Read the model definition and answer for the solid it produces. Units are mm, in the model's axes. A direction names the side the tool comes from. Coordinates: 2 decimals unless noted, no trailing zeros. Write each loop counter-clockwise with the first axis right and the second up, starting at its lowest first coordinate (ties: lowest second). Pieces come first, ordered by that corner, then holes.
Item 1: A tool of negligible diameter and unlimited length cuts with its end or side. For faces 4 (the face through (12.198, 8, 27)), 5 (the face through (47.427, 23, 19)), 6 (the face through (31.773, 19, 33)), from which of +Z, -Z, +X, -X, +Y, -Y can it reach the whole face along a straight path? Write none if from no direction.
Item 2: Section C-C (z = 17) is taken. Give the vertices of the cut face in (x, y), then the cut area to 3 significant figures.
Item 3: Each of these flat-tipped pins is pushed along its axis until it touches: P1, Ø3, axis at x = 38.5, z = 9, coming from the -Y side; P2, Ø4, axis at x = 36.5, y = 21.5, coming from the +Z side. Where does it stop, or does it pass through?
Item 4: Section D-D (y = 8) is taken. Give the vertices of the cut face in (x, z), then the cut area to 3 significant figures.
Item 5: Section A-A (z = 37) is taken. Give the vertices of the cut face in (x, y).
Item 6: Section B-B (x = 35.5) is taken. Give the vertices of the cut face in (y, z), then the cut area to 3 significant figures.
Item 7: Straight lines are drawn through the part: probe 1 along X at (y, z) = (35, 35.5); probe 2 along X at (y, z) = (6, 18.5); probe 3 along Z at (x, y) = (34, 29.5). For each, find the intervals that lie inside material, in ascending order.
Item 8: Determine the mould class of faces 1 (the face through (40.006, 19, 33)), 2 (the face through (12.198, 36, 27)), 3 (the face through (23, 45.912, 19)) for opening direction Y: released by +Y, released by -Y, zero draft, split by the parting line, or undercut.
from build123d import *

# Parameters (mm, degrees)
F0_W     = 47.427326
F0_H     = 45.911986
F1_DEPTH = 39.4099
F2_W     = 8.232169
F2_H     = 34.708312
F3_DEPTH = 13.71338
F5_DEPTH = 25.4


with BuildPart() as f1:
    # F0 (on Top) → F1 (new body)
    with BuildSketch(Plane.XY):
        with Locations((23.713663, 22.955993)):
            Rectangle(F0_W, F0_H)
    extrude(amount=F1_DEPTH)

    # F2 (on face) → F3 (cut)
    with BuildSketch(Plane.XY.offset(39.4099)):
        with Locations((35.889454, 19.653977)):
            Rectangle(F2_W, F2_H)
    extrude(amount=-F3_DEPTH, mode=Mode.SUBTRACT)

    # F4 (on face) → F5 (cut)
    with BuildSketch(Plane.XY.offset(39.4099)):
        with BuildLine():
            Line((12.198345, 45.911986), (12.198345, 25.47945))
            ThreePointArc((12.198345, 25.47945), (9.550043, 20.32), (12.198345, 15.16055))
            Line((12.198345, 15.16055), (12.198345, 0))
            Line((12.198345, 0), (19.601742, 0))
            Line((19.601742, 0), (19.601742, 15.16055))
            ThreePointArc((19.601742, 15.16055), (22.250043, 20.32), (19.601742, 25.47945))
            Line((19.601742, 25.47945), (19.601742, 45.911986))
            Line((19.601742, 45.911986), (12.198345, 45.911986))
        make_face()
    extrude(amount=-F5_DEPTH, mode=Mode.SUBTRACT)


solid = f1.part
Established:
1. face 4: +Z, +Y, -Y
1. face 5: +Z, -Z, +X, +Y, -Y
1. face 6: +Z
2. outline: (0, 0) - (12.2, 0) - (12.2, 15.16) arc R6.35 cw to (12.2, 25.48) - (12.2, 45.91) - (0, 45.91) - close; (19.6, 0) - (47.43, 0) - (47.43, 45.91) - (19.6, 45.91) - (19.6, 25.48) arc R6.35 cw to (19.6, 15.16) - close
2. area: 1,800 mm2
3. P1: stops at y = 0
3. P2: stops at z = 25.7
4. outline: (0, 0) - (47.43, 0) - (47.43, 39.41) - (40.01, 39.41) - (40.01, 25.7) - (31.77, 25.7) - (31.77, 39.41) - (19.6, 39.41) - (19.6, 14.01) - (12.2, 14.01) - (12.2, 39.41) - (0, 39.41) - close
4. area: 1,570 mm2
5. outline: (0, 0) - (12.2, 0) - (12.2, 15.16) arc R6.35 cw to (12.2, 25.48) - (12.2, 45.91) - (0, 45.91) - close; (19.6, 0) - (47.43, 0) - (47.43, 45.91) - (19.6, 45.91) - (19.6, 25.48) arc R6.35 cw to (19.6, 15.16) - close; hole (31.77, 2.3) - (40.01, 2.3) - (40.01, 37.01) - (31.77, 37.01) - close
6. outline: (0, 0) - (45.91, 0) - (45.91, 39.41) - (37.01, 39.41) - (37.01, 25.7) - (2.3, 25.7) - (2.3, 39.41) - (0, 39.41) - close
6. area: 1,330 mm2
7. probe 1: x = 0 to 12.2, 19.6 to 31.77, 40.01 to 47.43
7. probe 2: x = 0 to 12.2, 19.6 to 47.43
7. probe 3: z = 0 to 25.7
8. face 1: undercut
8. face 2: zero draft
8. face 3: released by +Y
